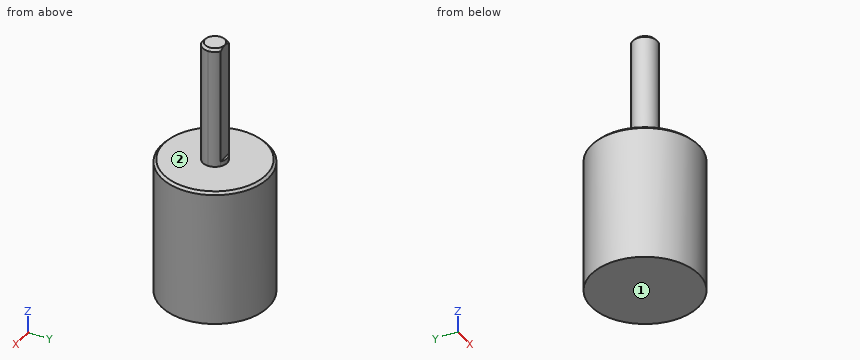
from build123d import *

# Parameters (mm, degrees)
SKETCH1_R           = 11
SKETCH1_R_2         = 2.5
BOSS_EXTRUDE1_DEPTH = 28
BOSS_EXTRUDE2_START = 28
BOSS_EXTRUDE2_DEPTH = 25
CUT_EXTRUDE1_START  = 29
CUT_EXTRUDE1_DEPTH  = 24
CHAMFER1_SIZE       = 0.5


with BuildPart() as part:
    # Sketch1 → Boss-Extrude1 (new body)
    # profile 1 of 5: a face of its own
    with BuildSketch(Plane.XY):
        Circle(SKETCH1_R)
        Circle(SKETCH1_R_2, mode=Mode.SUBTRACT)
    # profile 2 of 5: a face of its own
    with BuildSketch(Plane.XY):
        with BuildLine():
            ThreePointArc((1.5, 2), (0, 2.5), (-1.5, 2))
            Line((-1.5, 2), (1.5, 2))
        make_face()
    # profile 3 of 5: a face of its own
    with BuildSketch(Plane.XY):
        with BuildLine():
            Line((1.5, 2), (-1.5, 2))
            ThreePointArc((-1.5, 2), (-1.118033989, -2.236067977), (2.5, 0))
            ThreePointArc((2.5, 0), (2.236067977, 1.118033989), (1.5, 2))
        make_face()
    # profile 4 of 5: a face of its own
    with BuildSketch(Plane.XY):
        with BuildLine():
            ThreePointArc((1.5, 2), (0, 2.5), (-1.5, 2))
            Line((-1.5, 2), (1.5, 2))
        make_face()
    # profile 5 of 5: a face of its own
    with BuildSketch(Plane.XY):
        with BuildLine():
            Line((1.5, 2), (-1.5, 2))
            ThreePointArc((-1.5, 2), (-1.118033989, -2.236067977), (2.5, 0))
            ThreePointArc((2.5, 0), (2.236067977, 1.118033989), (1.5, 2))
        make_face()
    extrude(amount=BOSS_EXTRUDE1_DEPTH)

    # Sketch1<3> → Boss-Extrude2 (add)
    with BuildSketch(Plane.XY.offset(BOSS_EXTRUDE2_START)):
        with BuildLine():
            ThreePointArc((1.5, 2), (0, 2.5), (-1.5, 2))
            Line((-1.5, 2), (1.5, 2))
        make_face()
        with BuildLine():
            Line((1.5, 2), (-1.5, 2))
            ThreePointArc((-1.5, 2), (-1.118033989, -2.236067977), (2.5, 0))
            ThreePointArc((2.5, 0), (2.236067977, 1.118033989), (1.5, 2))
        make_face()
    extrude(amount=BOSS_EXTRUDE2_DEPTH)

    # Sketch1<4> → Cut-Extrude1 (cut)
    with BuildSketch(Plane.XY.offset(CUT_EXTRUDE1_START)):
        with BuildLine():
            ThreePointArc((1.5, 2), (0, 2.5), (-1.5, 2))
            Line((-1.5, 2), (1.5, 2))
        make_face()
    extrude(amount=CUT_EXTRUDE1_DEPTH, mode=Mode.SUBTRACT)

    # Chamfer1
    chamfer1_edges = [part.edges().sort_by_distance(p)[0] for p in [
        (-11, 0, 28),
        (-1.118033989, -2.236067977, 53),
    ]]
    chamfer(chamfer1_edges, length=CHAMFER1_SIZE - 0.0001)  # a hair under: the kernel refuses the full size


solid = part.part
CAD build for the part. Positions are in the model's coordinates, mm. Face numbers are marked on the shaded views. A direction names the side the tool comes from. Give positions to 0.01 mm unless a question says otherwise; leave off trailing zeros. Order: outer loops, then holes, each group sorted by start corner. A loop starts at its lowest first (then second) coordinate and runs counter-clockwise, first axis right, second up. Notation, with made-up numbers: (0.5, 65.25) -> (44.5, 65.25) arc R6 ccw to (44.5, 76.25) -> close; hole circle Ø6 at (88.25, 58.5). An arc over 180 degrees is marked (long way). Return JSON: item names as keys, results as strings.
Q1. Saw through at A-A (z = 28.5). Write the cut outline in (x, y), then the cut area to 3 significant figures.
Working result:
{"outline": "circle Ø5 at (0, 0)", "area": "19.6 mm²"}
Q2. Flat gauge pins, fed straight in: pin 1 (4 mm diameter, centred on y = 8.5, z = 21.5, fed in from +X); pin 2 (10 mm diameter, centred on x = 7, z = 19.5, fed in from -Y); pin 3 (1.5 mm diameter, centred on x = 0, z = 39, fed in from +Y). Where does each tip first touch, or does it go through?
Working result:
{"pin 1": "x = 8.87", "pin 2": "y = -10.82", "pin 3": "y = 2"}
Q3. Drill centre lines: line 1 (Z direction, x = 1.5, y = 6.5); line 2 (Y direction, x = 0.25, z = 33); line 3 (X direction, y = -6.25, z = 25). Where is each one in solid material? Low to high.
Working result:
{"line 1": "0 to 28", "line 2": "-2.49 to 2", "line 3": "-9.05 to 9.05"}
Q4. Which spindle directions (+Z, -Z, +X, -X, +Y, -Y) get a long thin tool onto all of the face, cutting with end or side? Do the marked faces 1 and 2. Say none if no direction does.
Working result:
{"face 1": "-Z, +X, -X, +Y, -Y", "face 2": "+Z"}
Q5. Saw through at B-B (z = 5.5). Write the cut outline in (x, y), then the cut area to 3 significant figures.
Working result:
{"outline": "circle Ø22 at (0, 0)", "area": "380 mm²"}
